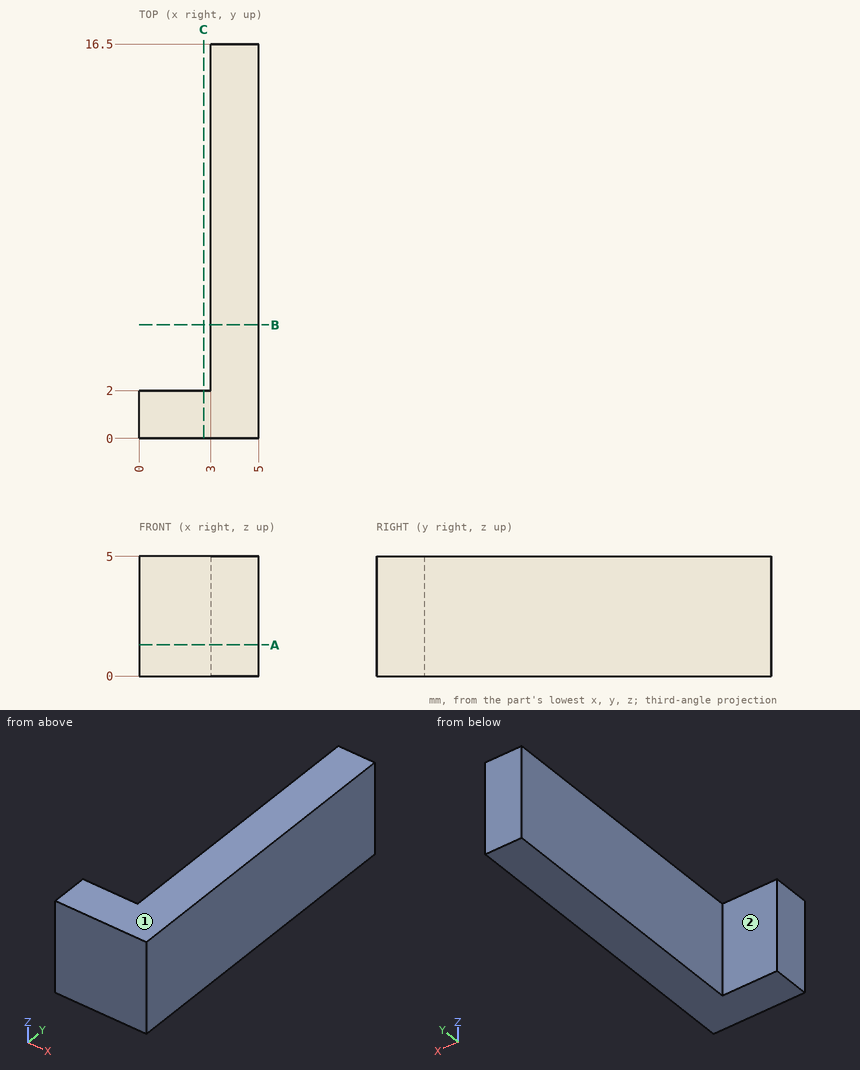
Print and shaded views of the part. All mm, measured from the part's lowest x, y and z. A direction names the side the tool comes from. Round coordinates to 2 decimals unless told otherwise and drop trailing zeros. Write each loop counter-clockwise with the first axis right and the second up, starting at its lowest first coordinate (ties: lowest second). Pieces come first, ordered by that corner, then holes. Notation, with made-up numbers: (-30, 34.5) -> (9, 34.5) arc R19 ccw to (9, 61.5) -> close; hole circle Ø10 at (24.5, 24.5). An arc over 180 degrees is marked (long way). Write item = value, one per line.
(1) Flat gauge pins, fed straight in: pin 1 (1.5 mm diameter, centred on y = 11.5, z = 3.5, fed in from -X); pin 2 (1.5 mm diameter, centred on x = 1.5, z = 1.5, fed in from +Y). Where does each tip first touch, or does it go through?
Answer:
pin_1 = 3
pin_2 = 2
(2) Band-saw the part on B-B (y = 4.75). Give the cut face in (x, z).
Answer:
outline = (3, 0) -> (5, 0) -> (5, 5) -> (3, 5) -> close
(3) Tool access for the marked faces 1 and 2: list every direction of +Z, -Z, +X, -X, +Y, -Y with a clear straight run to the whole face (end or side of a thin tool).
Answer:
face_1 = +Z, +X, -X, +Y, -Y
face_2 = +Z, -Z, -X, +Y
(4) Band-saw the part on C-C (x = 2.7). Give the cut face in (y, z), then the cut area to 3 significant figures.
Answer:
outline = (0, 0) -> (2, 0) -> (2, 5) -> (0, 5) -> close
area = 10.0 mm2
(5) Band-saw the part on A-A (z = 1.3). Give the cut face in (x, y), then the cut area to 3 significant figures.
Answer:
outline = (0, 0) -> (5, 0) -> (5, 16.5) -> (3, 16.5) -> (3, 2) -> (0, 2) -> close
area = 39.0 mm2
(6) Probe L1, parallel to X at y = 12, z = 4.75; L2, parallel to Y at x = 1.1, z = 3.5. List the from-to ranges inside material, lowest first.
Answer:
L1 = 3 to 5
L2 = 0 to 2
